Part model, mm, in its own coordinate system. Face numbers are marked on the shaded views. A direction names the side the tool comes from. Give positions to 0.01 mm unless a question says otherwise; leave off trailing zeros. Order: outer loops, then holes, each group sorted by start corner. A loop starts at its lowest first (then second) coordinate and runs counter-clockwise, first axis right, second up. Notation, with made-up numbers: (34.25, 88) -> (59.25, 88) arc R32 ccw to (59.25, 120) -> close; hole circle Ø9 at (38.25, 33.25). An arc over 180 degrees is marked (long way). Write item = value, one per line. Start each with the question number.
Item 1: Band-saw the part on C-C on y = -7.5. Write the cut outline in (x, z), plus the area to 3 significant figures.
Item 2: Pull direction X, two halves, no side cores. Call the marked faces 4, 5 and 6: +X half, -X half, draft (parallel to the pull), parting line (faces both ways), or undercut.
Item 3: Band-saw the part on B-B on x = 0. Write the cut outline in (y, z), plus the area to 3 significant figures.
Item 4: Band-saw the part on A-A on y = -89. Write the cut outline in (x, z), plus the area to 3 significant figures.
Item 5: Flat gauge pins, fed straight in: P1, Ø2, axis at x = -29.5, y = -33, coming from the +Z side; P2, Ø8, axis at x = -19, y = -29.5, coming from the -Z side; P3, Ø10, axis at x = -26.5, y = -54, coming from the +Z side; P4, Ø1.5, axis at y = -81.5, z = -2.5, coming from the -X side. Where does each tip first touch, or does it go through?
Item 6: Tool access for the marked faces 1, 2 and 3: list every direction of +Z, -Z, +X, -X, +Y, -Y with a clear straight run to the whole face (end or side of a thin tool).
Item 7: Drill centre lines: line 1 along X through (y, z) = (-66.5, -17.5); line 2 along Z through (x, y) = (36, -41.5); line 3 along Y through (x, z) = (4.5, 5). Where is each one in solid material? Low to high.
```python
from build123d import *

# Parameters (mm, degrees)
SKETCH2_W           = 12.7
SKETCH2_H           = 5.158072601
BOSS_EXTRUDE1_DEPTH = 30.48
BOSS_EXTRUDE2_DEPTH = 6.35


with BuildPart() as part:
    # Sketch1 → Revolve1 (revolve)
    with BuildSketch(Plane.XY, mode=Mode.PRIVATE) as revolve1_sk:
        with BuildLine():
            Line((5.497877947, -31.389690294), (5.282120164, -24.249424513))
            ThreePointArc((5.282120164, -24.249424513), (12.409022752, -9.99701011), (0, 0))
            Line((0, 0), (0, -70.812800241))
            Line((0, -70.812800241), (36.63136247, -70.812800241))
            Line((36.63136247, -70.812800241), (5.497877947, -31.389690294))
        make_face()
    revolve(revolve1_sk.sketch.rotate(Axis((0, 0, 0), (0, -1, 0)), 90), axis=Axis((0, 0, 0), (0, -1, 0)))  # turned: the seam where the file's is

    # Sketch2 → Boss-Extrude1 (add)
    with BuildSketch(Plane(origin=(0, -70.812800241, 0), x_dir=(-1, 0, 0), z_dir=(0, -1, 0))):
        with Locations((13.97, -2.5009637)):
            Rectangle(SKETCH2_W, SKETCH2_H)
        with Locations((-13.97, 2.5009637)):
            Rectangle(SKETCH2_W, SKETCH2_H)
    extrude(amount=BOSS_EXTRUDE1_DEPTH)

    # Sketch4 → Boss-Extrude2 (add, symmetric)
    with BuildSketch(Plane.XY.offset(2.54)):
        with BuildLine():
            Line((23.194397658, -58.195407075), (28.218678504, -58.195407075))
            ThreePointArc((28.218678504, -58.195407075), (30.027441839, -57.44619277), (31.836205173, -58.195407075))
            ThreePointArc((31.836205173, -58.195407075), (34.251957858, -57.421245639), (36.286043383, -58.937056657))
            ThreePointArc((36.286043383, -58.937056657), (38.347997753, -58.082967192), (40.409952123, -58.937056657))
            ThreePointArc((40.409952123, -58.937056657), (42.564346856, -57.773722125), (44.910335716, -58.474507515))
            ThreePointArc((44.910335716, -58.474507515), (45.361627038, -57.049665796), (44.673222951, -55.723039401))
            ThreePointArc((44.673222951, -55.723039401), (45.573759248, -53.584134002), (44.698100059, -51.434924167))
            ThreePointArc((44.698100059, -51.434924167), (45.526766993, -49.466398887), (44.720765428, -47.488485304))
            ThreePointArc((44.720765428, -47.488485304), (45.146776163, -45.049852477), (43.723637436, -43.024243586))
            ThreePointArc((43.723637436, -43.024243586), (44.720765428, -41.476171224), (44.331188928, -39.676442795))
            ThreePointArc((44.331188928, -39.676442795), (44.916218335, -36.976008484), (43.420401182, -34.652834811))
            ThreePointArc((43.420401182, -34.652834811), (43.980987953, -32.721408857), (43.01165827, -30.959289761))
            ThreePointArc((43.01165827, -30.959289761), (43.155496077, -29.184392296), (42.002162733, -27.827641575))
            Line((42.002162733, -27.827641575), (45.598003191, -22.653559314))
            Line((45.598003191, -22.653559314), (43.420401182, -23.871865995))
            ThreePointArc((43.420401182, -23.871865995), (40.913084014, -23.73552357), (39.043734388, -25.41205589))
            ThreePointArc((39.043734388, -25.41205589), (37.052487537, -25.435932109), (35.661346423, -26.860839296))
            ThreePointArc((35.661346423, -26.860839296), (33.825367945, -27.399752632), (32.908204388, -29.079054738))
            ThreePointArc((32.908204388, -29.079054738), (31.003426578, -28.874097378), (29.511618532, -30.076051946))
            ThreePointArc((29.511618532, -30.076051946), (27.807974314, -31.448683603), (27.573913087, -33.623939136))
            ThreePointArc((27.573913087, -33.623939136), (25.608192785, -33.412424259), (24.068655026, -34.652834811))
            ThreePointArc((24.068655026, -34.652834811), (21.607314855, -35.264896302), (20.299677359, -37.438119458))
            ThreePointArc((20.299677359, -37.438119458), (18.321683781, -37.929987145), (17.270834086, -39.676442795))
            Line((17.270834086, -39.676442795), (12.250540769, -43.386453078))
            Line((12.250540769, -43.386453078), (23.194397658, -58.195407075))
        make_face()
        with BuildLine():
            Line((-23.194397658, -58.195407075), (-28.218678504, -58.195407075))
            ThreePointArc((-28.218678504, -58.195407075), (-30.027441839, -57.44619277), (-31.836205173, -58.195407075))
            ThreePointArc((-31.836205173, -58.195407075), (-34.251957858, -57.421245639), (-36.286043383, -58.937056657))
            ThreePointArc((-36.286043383, -58.937056657), (-38.347997753, -58.082967192), (-40.409952123, -58.937056657))
            ThreePointArc((-40.409952123, -58.937056657), (-42.564346856, -57.773722125), (-44.910335716, -58.474507515))
            ThreePointArc((-44.910335716, -58.474507515), (-45.361627038, -57.049665796), (-44.673222951, -55.723039401))
            ThreePointArc((-44.673222951, -55.723039401), (-45.573759248, -53.584134002), (-44.698100059, -51.434924167))
            ThreePointArc((-44.698100059, -51.434924167), (-45.526766993, -49.466398887), (-44.720765428, -47.488485304))
            ThreePointArc((-44.720765428, -47.488485304), (-45.146776163, -45.049852477), (-43.723637436, -43.024243586))
            ThreePointArc((-43.723637436, -43.024243586), (-44.720765428, -41.476171224), (-44.331188928, -39.676442795))
            ThreePointArc((-44.331188928, -39.676442795), (-44.916218335, -36.976008484), (-43.420401182, -34.652834811))
            ThreePointArc((-43.420401182, -34.652834811), (-43.980987953, -32.721408857), (-43.01165827, -30.959289761))
            ThreePointArc((-43.01165827, -30.959289761), (-43.155496077, -29.184392296), (-42.002162733, -27.827641575))
            Line((-42.002162733, -27.827641575), (-45.598003191, -22.653559314))
            Line((-45.598003191, -22.653559314), (-43.420401182, -23.871865995))
            ThreePointArc((-43.420401182, -23.871865995), (-40.913084014, -23.73552357), (-39.043734388, -25.41205589))
            ThreePointArc((-39.043734388, -25.41205589), (-37.052487537, -25.435932109), (-35.661346423, -26.860839296))
            ThreePointArc((-35.661346423, -26.860839296), (-33.825367945, -27.399752632), (-32.908204388, -29.079054738))
            ThreePointArc((-32.908204388, -29.079054738), (-31.003426578, -28.874097378), (-29.511618532, -30.076051946))
            ThreePointArc((-29.511618532, -30.076051946), (-27.807974314, -31.448683603), (-27.573913087, -33.623939136))
            ThreePointArc((-27.573913087, -33.623939136), (-25.608192785, -33.412424259), (-24.068655026, -34.652834811))
            ThreePointArc((-24.068655026, -34.652834811), (-21.607314855, -35.264896302), (-20.299677359, -37.438119458))
            ThreePointArc((-20.299677359, -37.438119458), (-18.321683781, -37.929987145), (-17.270834086, -39.676442795))
            Line((-17.270834086, -39.676442795), (-12.250540769, -43.386453078))
            Line((-12.250540769, -43.386453078), (-23.194397658, -58.195407075))
        make_face()
    extrude(amount=BOSS_EXTRUDE2_DEPTH, both=True)


solid = part.part
```
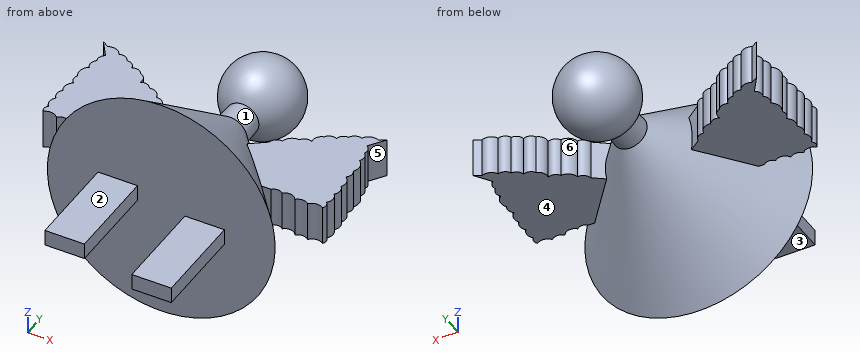
Values found:
q1.outline = circle Ø23.17 at (0, 0)
q1.area = 422 mm^2
q2.face_4 = draft
q2.face_5 = +X half
q2.face_6 = undercut
q3.outline = (-70.81, -36.63) -> (-31.39, -5.5) -> (-24.25, -5.28) arc R12.7 ccw (long way) to (-24.25, 5.28) -> (-31.39, 5.5) -> (-70.81, 36.63) -> close
q3.area = 2,240 mm^2
q4.outline = (-20.32, -0.08) -> (-7.62, -0.08) -> (-7.62, 5.08) -> (-20.32, 5.08) -> close; (7.62, -5.08) -> (20.32, -5.08) -> (20.32, 0.08) -> (7.62, 0.08) -> close
q4.area = 131 mm^2
q5.P1 = 8.89
q5.P2 = through
q5.P3 = 12.52
q5.P4 = 7.62
q6.face_1 = none
q6.face_2 = +Z, +X, -X, -Y
q6.face_3 = -Z, -X, -Y
q7.line_1 = -28.24 to 28.24
q7.line_2 = -3.81 to 8.89
q7.line_3 = -70.81 to -32.95, -23.47 to -1.93
